Model file for the job. Use its own axes, mm. Face numbers are marked on the shaded views. A direction names the side the tool comes from. Give positions to 0.01 mm unless a question says otherwise; leave off trailing zeros. Loops run counter-clockwise (first coordinate to the right, second up) from the corner with the lowest first, then second, coordinate; pieces in that order, holes last. Notation, with made-up numbers: (-6.75, 2.5) - (3.25, 2.5) arc R29 ccw to (3.25, 26.5) - close; hole circle Ø2 at (-3, 42.5). An arc over 180 degrees is marked (long way). Use a Markdown table: item, result.
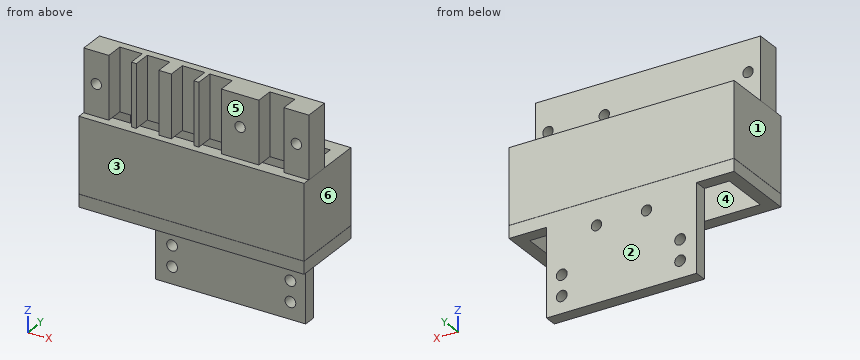
from build123d import *

# Parameters (mm, degrees)
F1_DEPTH  = 25
F2_W      = 90
F2_H      = 30
F2_W_2    = 79.8000005633
F2_H_2    = 19.8000005633
F3_DEPTH  = 30
F5_W      = 90
F5_H      = 30
F6_DEPTH  = 5
F7_W      = 60
F7_H      = 5
F8_DEPTH  = 35
F9_R      = 2.075
F10_DEPTH = 5
F12_R     = 2.075
F13_DEPTH = 10
F15_R     = 2.15
F16_DEPTH = 5
F17_DEPTH = 35


with BuildPart() as f1:
    # F0 (on Top) → F1 (new body)
    with BuildSketch(Plane.XY):
        Polygon((-20, 0), (-45, 0), (-45, -10), (-35, -10), (-35, -3), (-26, -3), (-26, -10), (-24, -10.0096508846), (-24, -3), (-15, -3), (-15, -10), (-10, -10), (-10, -3), (-1, -3), (-1, -10), (1, -10), (1, -3), (10, -3), (10, -10), (25, -10), (25, -3), (35, -3), (35, -10), (45, -10), (45, 0), (20, 0), align=None)
    extrude(amount=F1_DEPTH)

    # F2 (on Top) → F3 (join)
    with BuildSketch(Plane.XY):
        with Locations((-0.0773276389, 2.026154995)):
            Rectangle(F2_W, F2_H)
        with Locations((-0.0773276389, 2.026154995)):
            Rectangle(F2_W_2, F2_H_2, mode=Mode.SUBTRACT)
    extrude(amount=-F3_DEPTH)

    # F5 (on offset) → F6 (join)
    with BuildSketch(Plane(origin=(0, 0, -30), x_dir=(1, 0, 0), z_dir=(0, 0, -1))):
        with Locations((-0.0007246435, -1.9418361038)):
            Rectangle(F5_W, F5_H)
    extrude(amount=F6_DEPTH)

    # F7 (on face) → F8 (join)
    with BuildSketch(Plane(origin=(0, 0, -35), x_dir=(1, 0, 0), z_dir=(0, 0, -1))):
        with Locations((-0.0007246435, -14.4418361038)):
            Rectangle(F7_W, F7_H)
    extrude(amount=F8_DEPTH)

    # F9 (on face) → F10 (cut, through all)
    with BuildSketch(Plane.XZ.offset(-11.9418361038)):
        with Locations((-10.0007246435, -40)):
            Circle(F9_R)
        with Locations((9.9992753565, -40)):
            Circle(F9_R)
    extrude(amount=-F10_DEPTH, mode=Mode.SUBTRACT)

    # F12 (on offset) → F13 (cut, through all)
    with BuildSketch(Plane(origin=(0, -10, 0), x_dir=(-1, 0, 0), z_dir=(0, 1, 0))):
        with Locations((40, 12.5)):
            Circle(F12_R)
        with Locations((-17.5, 12.5)):
            Circle(F12_R)
        with Locations((-40, 12.5)):
            Circle(F12_R)
    extrude(amount=F13_DEPTH, mode=Mode.SUBTRACT)

    # F15 (on offset) → F16 (cut, through all)
    with BuildSketch(Plane(origin=(0, 16.9418361038, 0), x_dir=(-1, 0, 0), z_dir=(0, 1, 0))):
        with Locations((23.4303546713, -55.0644522592)):
            Circle(F15_R)
        with Locations((-23.8896453287, -55.0644522592)):
            Circle(F15_R)
        with Locations((-23.8896453287, -63.2644522592)):
            Circle(F15_R)
        with Locations((23.4303546713, -63.2644522592)):
            Circle(F15_R)
    extrude(amount=-F16_DEPTH, mode=Mode.SUBTRACT)

    # F2 (on Top) → F17 (cut)
    with BuildSketch(Plane.XY):
        with Locations((-0.0773276389, 2.026154995)):
            Rectangle(F2_W_2, F2_H_2)
    extrude(amount=-F17_DEPTH, mode=Mode.SUBTRACT)


solid = f1.part
(1) Slice it at A-A, the plane x = 32. Write the cut outline in (y, z).
Computed:
| item | result |
|---|---|
| outline | (-13.06, -35) - (-7.87, -35) - (-7.87, 0) - (-12.97, 0) - (-12.97, -30) - (-13.06, -30) - close; (-3, 0) - (0, 0) - (0, 25) - (-3, 25) - close; (11.93, -35) - (16.94, -35) - (16.94, -30) - (17.03, -30) - (17.03, 0) - (11.93, 0) - close |
(2) Drill centre lines: probe 1 along Y at (x, z) = (26, -0.5); probe 2 along X at (y, z) = (-7.5, -5.5); probe 3 along Y at (x, z) = (21, -31.5). Where is each one in solid material? Low to high. Write a range as [from, to].
Computed:
| item | result |
|---|---|
| probe 1 | [-12.97, -7.87], [11.93, 17.03] |
| probe 2 | [-45.08, -39.98], [39.82, 44.92] |
| probe 3 | [-13.06, -7.87], [11.93, 16.94] |
(3) Slice it at B-B, the plane z = -40. Write the cut outline in (x, y).
Computed:
| item | result |
|---|---|
| outline | (-30, 11.94) - (-12.08, 11.94) - (-12.08, 16.94) - (-30, 16.94) - close; (-7.93, 11.94) - (7.92, 11.94) - (7.92, 16.94) - (-7.93, 16.94) - close; (12.07, 11.94) - (30, 11.94) - (30, 16.94) - (12.07, 16.94) - close |
(4) Slice it at C-C, the plane y = -5. Count the separate pieces of the cut face and the enclosed holes in it, plus the area to 3 significant figures.
Computed:
| item | result |
|---|---|
| separate pieces | 6 |
| enclosed holes | 3 |
| area | 1,420 mm² |
(5) Pin check, flat tips, straight feed: P1, Ø3.5, axis at x = -40, z = 12.5, coming from the -Y side; P2, Ø3, axis at x = 28.5, z = 16.5, coming from the -Y side; P3, Ø7.5, axis at y = -6.5, z = 13, coming from the -X side; P4, Ø8, axis at x = 35.5, y = -6, coming from the -Z side. Stop position of each tip, or through.
Computed:
| item | result |
|---|---|
| P1 | through |
| P2 | y = -3 |
| P3 | x = -45 |
| P4 | z = -35 |
(6) 3-axis set-ups, long thin cutter, end or side, ignore diameter. For the marked faces 1, 2 and 3: which of +Z, -Z, +X, -X, +Y, -Y reach the whole face in a straight line?
Computed:
| item | result |
|---|---|
| face 1 | +Z, -Z, -X, +Y, -Y |
| face 2 | -Z, +X, -X, +Y |
| face 3 | +Z, +X, -X, -Y |
(7) Mould opens along X. For the marked faces 4, 5 and 6 say: pulls with the +X half, pulls with the -X half, needs draft (parallel to the pull), parting line crosses it, or undercut.
Computed:
| item | result |
|---|---|
| face 4 | undercut |
| face 5 | needs draft |
| face 6 | pulls with the +X half |
(8) Slice it at D-D, the plane z = -28.5. Write the cut outline in (x, y), plus the area to 3 significant figures.
Computed:
| item | result |
|---|---|
| outline | (-45.08, -12.97) - (44.92, -12.97) - (44.92, 17.03) - (-45.08, 17.03) - close; hole (-39.98, -7.87) - (39.82, -7.87) - (39.82, 11.93) - (-39.98, 11.93) - close |
| area | 1,120 mm² |
